Geometry check sheet. Reference: the model listing, model coordinates, mm. Face numbers are marked on the shaded views. Coordinates: 2 decimals unless noted, no trailing zeros. Write each loop counter-clockwise with the first axis right and the second up, starting at its lowest first coordinate (ties: lowest second). Pieces come first, ordered by that corner, then holes. Notation, with made-up numbers: (-3, -22.75) -> (54, -22.75) arc R16 ccw to (54, -16.75) -> close; hole circle Ø8 at (-7.75, -33.75). An arc over 180 degrees is marked (long way). Answer in a Markdown table with one row per item. Add a question column.
Q1. Section check B-B, the plane z = 2.25. Record the boundary of the cut face in (x, y), and give its area (3 significant figures).
Q2. Thickness scan on line 1 (Y direction, x = 0, z = 2.7); line 2 (X direction, y = 0.25, z = 3); line 3 (Y direction, x = -0.5, z = 1.85). Record the ranges inside material, lowest first.
Q3. Section check C-C, the plane y = 3.25. Record the boundary of the cut face in (x, z).
Q4. Release check for a two-part mould opening along X. For the marked faces 1, 2 and 3 record: pulls with the +X half, pulls with the -X half, needs draft (parallel to the pull), parting line crosses it, or undercut.
Q5. Section check A-A, the plane x = 0. Record the boundary of the cut face in (y, z).
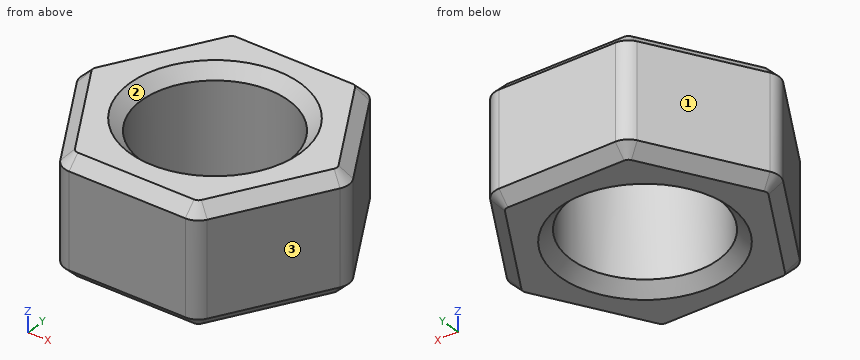
Autodesk Inventor part; units mm, degrees
ref_plane "YZ Plane" through (0, 0, 0) normal (1, 0, 0) x (0, 1, 0)
ref_plane "XZ Plane" through (0, 0, 0) normal (0, 1, 0) x (-1, 0, 0)
ref_plane "XY Plane" through (0, 0, 0) normal (0, 0, 1) x (1, 0, 0)
sketch "Эскиз1" plane through (0, 0, 0) normal (0, 0, 1) x (1, 0, 0)
  circle A0 centre (0, 0) radius 2.5
  line L0 (2.3094, 4) -> (4.6188, 0)
  line L1 (4.6188, 0) -> (2.3094, -4)
  line L2 (2.3094, -4) -> (-2.3094, -4)
  line L3 (-2.3094, -4) -> (-4.6188, 0)
  line L4 (-4.6188, 0) -> (-2.3094, 4)
  line L5 (-2.3094, 4) -> (2.3094, 4)
  dimension "d0" = 5
  dimension "d1" = 8
extrude "Выдавливание1" add sketch "Эскиз1" along normal blind 4
fillet "Сопряжение1" radius 0.6 6 edges at (-4.6188, 0, 2) (-2.3094, -4, 2) (2.3094, -4, 2) (4.6188, 0, 2) (2.3094, 4, 2) (-2.3094, 4, 2)
chamfer "Фаска1" distance 0.4 angle 45 26 edges at (0, 4, 0) (-2.263, 3.9196, 0) (-3.4641, 2, 0) (-4.526, 0, 0) (-3.4641, -2, 0) (-2.263, -3.9196, 0) (0, -4, 0) (2.263, -3.9196, 0) (3.4641, -2, 0) (4.526, 0, 0) (3.4641, 2, 0) (2.263, 3.9196, 0) (0, 4, 4) (-2.263, 3.9196, 4) (-3.4641, 2, 4) (-4.526, 0, 4) (-3.4641, -2, 4) (-2.263, -3.9196, 4) (0, -4, 4) (2.263, -3.9196, 4) (3.4641, -2, 4) (4.526, 0, 4) (3.4641, 2, 4) (2.263, 3.9196, 4) (-2.5, 0, 4) (-2.5, 0, 0)
properties part number "Гайка М5"
Calculated:
| question | item | result |
|---|---|---|
| 1 | outline | (-4.45, -0.3) -> (-2.48, -3.7) arc R0.6 ccw to (-1.96, -4) -> (1.96, -4) arc R0.6 ccw to (2.48, -3.7) -> (4.45, -0.3) arc R0.6 ccw to (4.45, 0.3) -> (2.48, 3.7) arc R0.6 ccw to (1.96, 4) -> (-1.96, 4) arc R0.6 ccw to (-2.48, 3.7) -> (-4.45, 0.3) arc R0.6 ccw to start; hole circle Ø5 at (0, 0) |
| 1 | area | 35.7 mm² |
| 2 | line 1 | y = -4 to -2.5, 2.5 to 4 |
| 2 | line 2 | x = -4.47 to -2.49, 2.49 to 4.47 |
| 2 | line 3 | y = -4 to -2.45, 2.45 to 4 |
| 3 | outline | (-2.74, 0.4) -> (-2.28, 0) -> (2.28, 0) -> (2.74, 0.4) -> (2.74, 3.6) -> (2.28, 4) -> (-2.28, 4) -> (-2.74, 3.6) -> close |
| 4 | face 1 | pulls with the -X half |
| 4 | face 2 | undercut |
| 4 | face 3 | pulls with the +X half |
| 5 | outline | (-4, 0.4) -> (-3.6, 0) -> (-2.9, 0) -> (-2.5, 0.4) -> (-2.5, 3.6) -> (-2.9, 4) -> (-3.6, 4) -> (-4, 3.6) -> close; (2.5, 0.4) -> (2.9, 0) -> (3.6, 0) -> (4, 0.4) -> (4, 3.6) -> (3.6, 4) -> (2.9, 4) -> (2.5, 3.6) -> close |
